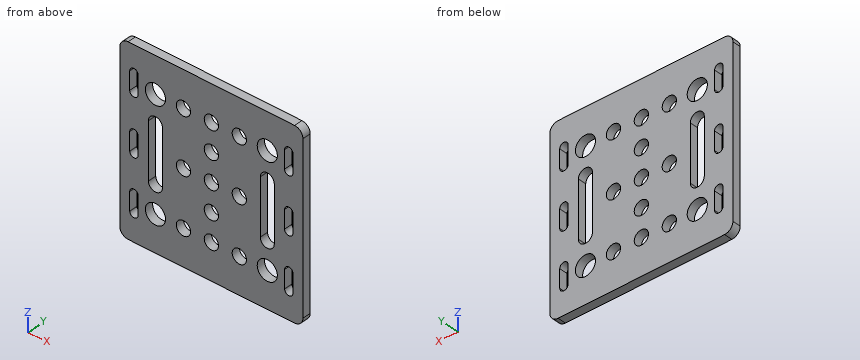
Autodesk Inventor part; units mm, degrees
ref_plane "YZ Plane" through (0, 0, 0) normal (1, 0, 0) x (0, 1, 0)
ref_plane "XZ Plane" through (0, 0, 0) normal (0, 1, 0) x (-1, 0, 0)
ref_plane "XY Plane" through (0, 0, 0) normal (0, 0, 1) x (1, 0, 0)
sketch "Sketch1" plane through (0, 0, 0) normal (0, 1, 0) x (-1, 0, 0)
  line L0 (-29.75, 32.75) -> (29.75, 32.75)
  line L1 (32.75, 29.75) -> (32.75, -29.75)
  line L2 (29.75, -32.75) -> (-29.75, -32.75)
  line L3 (-32.75, -29.75) -> (-32.75, 29.75)
  arc A0 (-29.75, 32.75) -> (-32.75, 29.75) centre (-29.75, 29.75) ccw
  arc A1 (-32.75, -29.75) -> (-29.75, -32.75) centre (-29.75, -29.75) ccw
  arc A2 (29.75, -32.75) -> (32.75, -29.75) centre (29.75, -29.75) ccw
  arc A3 (32.75, 29.75) -> (29.75, 32.75) centre (29.75, 29.75) ccw
  arc A4 (29.2, 23.4) -> (26.2, 23.4) centre (27.7, 23.4) ccw
  arc A5 (26.2, 16.9) -> (29.2, 16.9) centre (27.7, 16.9) ccw
  line L4 (29.2, 23.4) -> (29.2, 16.9)
  line L5 (26.2, 23.4) -> (26.2, 16.9)
  arc A6 (29.2, 3.25) -> (26.2, 3.25) centre (27.7, 3.25) ccw
  arc A7 (26.2, -3.25) -> (29.2, -3.25) centre (27.7, -3.25) ccw
  line L6 (29.2, 3.25) -> (29.2, -3.25)
  line L7 (26.2, 3.25) -> (26.2, -3.25)
  circle A8 centre (20, 19.85) radius 3.6
  circle A9 centre (10, 19.85) radius 2.55
  circle A10 centre (0, 19.85) radius 2.55
  circle A11 centre (0, 10) radius 2.55
  circle A12 centre (0, 0) radius 2.55
  circle A13 centre (10, 0) radius 2.55
  arc A14 (22.5, 10) -> (17.5, 10) centre (20, 10) ccw
  arc A15 (17.5, -10) -> (22.5, -10) centre (20, -10) ccw
  line L8 (22.5, 10) -> (22.5, -10)
  line L9 (17.5, 10) -> (17.5, -10)
  circle A16 centre (-20, 19.85) radius 3.6
  circle A17 centre (20, -19.85) radius 3.6
  circle A18 centre (-20, -19.85) radius 3.6
  circle A19 centre (-10, 19.85) radius 2.55
  circle A20 centre (-10, -19.85) radius 2.55
  circle A21 centre (10, -19.85) radius 2.55
  circle A22 centre (0, -10) radius 2.55
  circle A23 centre (0, -19.85) radius 2.55
  circle A24 centre (-10, 0) radius 2.55
  arc A25 (-17.5, 10) -> (-22.5, 10) centre (-20, 10) ccw
  arc A26 (-22.5, -10) -> (-17.5, -10) centre (-20, -10) ccw
  line L10 (-17.5, 10) -> (-17.5, -10)
  line L11 (-22.5, 10) -> (-22.5, -10)
  arc A27 (29.2, -16.6) -> (26.2, -16.6) centre (27.7, -16.6) ccw
  arc A28 (26.2, -23.1) -> (29.2, -23.1) centre (27.7, -23.1) ccw
  line L12 (29.2, -16.6) -> (29.2, -23.1)
  line L13 (26.2, -16.6) -> (26.2, -23.1)
  line L14 (-32.75, 32.75) -> (-27.7, 32.75)
  arc A29 (-26.2, 23.1) -> (-29.2, 23.1) centre (-27.7, 23.1) ccw
  arc A30 (-29.2, 16.6) -> (-26.2, 16.6) centre (-27.7, 16.6) ccw
  line L15 (-26.2, 23.1) -> (-26.2, 16.6)
  line L16 (-29.2, 23.1) -> (-29.2, 16.6)
  arc A31 (-26.2, 3.25) -> (-29.2, 3.25) centre (-27.7, 3.25) ccw
  arc A32 (-29.2, -3.25) -> (-26.2, -3.25) centre (-27.7, -3.25) ccw
  line L17 (-26.2, 3.25) -> (-26.2, -3.25)
  line L18 (-29.2, 3.25) -> (-29.2, -3.25)
  arc A33 (-26.2, -16.6) -> (-29.2, -16.6) centre (-27.7, -16.6) ccw
  arc A34 (-29.2, -23.1) -> (-26.2, -23.1) centre (-27.7, -23.1) ccw
  line L19 (-26.2, -16.6) -> (-26.2, -23.1)
  line L20 (-29.2, -16.6) -> (-29.2, -23.1)
  point P0 (0, 0)
  point P1 (27.7, 0)
  point P2 (-27.7, 19.85)
  point P3 (-27.7, 0)
  point P4 (-27.7, -19.85)
  dimension "d2" = 3
  dimension "d7" = 3
  dimension "d8" = 3
  dimension "d10" = 3
  dimension "d12" = 3
  dimension "d16" = 7.2
  dimension "d18" = 5.1
  dimension "d20" = 5.1
  dimension "d22" = 5.1
  dimension "d23" = 5.1
  dimension "d24" = 5.1
  dimension "d26" = 5
  dimension "d28" = 5
  dimension "d31" = 10
  dimension "d36" = 7.2
  dimension "d39" = 29.5
  dimension "d44" = 7.2
  dimension "d45" = 7.2
  dimension "d46" = 5.1
  dimension "d47" = 5.1
  dimension "d48" = 5.1
  dimension "d51" = 5.1
  dimension "d52" = 5.1
  dimension "d53" = 5.1
  dimension "d54" = 5
  dimension "d55" = 5
  dimension "d56" = 3
  dimension "d57" = 3
  dimension "d58" = 5.05
  dimension "d59" = 3
  dimension "d60" = 3
  dimension "d61" = 3
  dimension "d62" = 3
  dimension "d63" = 3
  dimension "d64" = 3
extrude "Extrusion1" add sketch "Sketch1" along normal blind 3
properties part number "Plataforma"
Read the model definition and answer for the solid it produces. Units are mm, in the model's axes. Coordinates: 2 decimals unless noted, no trailing zeros. Loops run counter-clockwise (first coordinate to the right, second up) from the corner with the lowest first, then second, coordinate; pieces in that order, holes last. Notation, with made-up numbers: (-33, 14.5) -> (14, 14.5) arc R10 ccw to (14, 23.5) -> close; hole circle Ø11 at (17.25, 54). An arc over 180 degrees is marked (long way). Return JSON: item names as keys, results as strings.
Item 1: Find the intervals of material crossed by probe 1 along Z at (x, y) = (0, 0.85); probe 2 along Z at (x, y) = (-20, 0.95); probe 3 along Z at (x, y) = (10, 2.45), in increasing order.
Answers:
{"probe 1": "z = -32.75 to -22.4, -17.3 to -12.55, -7.45 to -2.55, 2.55 to 7.45, 12.55 to 17.3, 22.4 to 32.75", "probe 2": "z = -32.75 to -23.45, -16.25 to -12.5, 12.5 to 16.25, 23.45 to 32.75", "probe 3": "z = -32.75 to -22.4, -17.3 to -2.55, 2.55 to 17.3, 22.4 to 32.75"}
Item 2: Find section B-B (z = 0). Count the separate pieces of the cut face and the enclosed holes in it, plus the area to 3 significant figures.
Answers:
{"separate pieces": "8", "enclosed holes": "0", "area": "103 mm2"}
Item 3: Find section C-C (x = -27.7). Determine the outline of the cut face in (y, z).
Answers:
{"outline": "(0, -32.75) -> (3, -32.75) -> (3, -24.6) -> (0, -24.6) -> close; (0, -15.1) -> (3, -15.1) -> (3, -4.75) -> (0, -4.75) -> close; (0, 4.75) -> (3, 4.75) -> (3, 15.4) -> (0, 15.4) -> close; (0, 24.9) -> (3, 24.9) -> (3, 32.75) -> (0, 32.75) -> close"}
Item 4: Find section A-A (x = -20). Determine the outline of the cut face in (y, z), plus the area to 3 significant figures.
Answers:
{"outline": "(0, -32.75) -> (3, -32.75) -> (3, -23.45) -> (0, -23.45) -> close; (0, -16.25) -> (3, -16.25) -> (3, -12.5) -> (0, -12.5) -> close; (0, 12.5) -> (3, 12.5) -> (3, 16.25) -> (0, 16.25) -> close; (0, 23.45) -> (3, 23.45) -> (3, 32.75) -> (0, 32.75) -> close", "area": "78.3 mm2"}
